from build123d import *

# Parameters (mm, degrees)
BOSS_EXTRUDE1_DEPTH     = 38.1
SKETCH2_W               = 25.4
SKETCH2_H               = 31.75
CUT_EXTRUDE1_DEPTH      = 88.9
CUT_EXTRUDE2_REACH      = 133.37
SKETCH3_W               = 25.4
SKETCH3_H               = 31.75
CUT_EXTRUDE3_START      = -62.861793
SKETCH4_W               = 75
SKETCH4_H               = 31.75
CUT_EXTRUDE3_DEPTH      = 28.575
FILLET4_R               = 20
CUT_EXTRUDE8_DEPTH      = 131.484388453
CUT_EXTRUDE8_DEPTH_BACK = 131.484388453
SKETCH8_R               = 6.35
BOSS_EXTRUDE2_DEPTH     = 3.175
CUT_EXTRUDE10_REACH     = 133.37
SKETCH35_R              = 3.175
CUT_EXTRUDE11_REACH     = 133.37
SKETCH36_R              = 3.175
FILLET8_R               = 5
CHAMFER1_SIZE           = 10
CHAMFER1_SIZE_2         = 7.071067812
CUT_EXTRUDE12_REACH     = 133.37
SKETCH37_R              = 3.175


with BuildPart() as part:
    # Sketch1 → Boss-Extrude1 (new body)
    with BuildSketch(Plane(origin=(0, 0, 0), x_dir=(1, 0, 0), z_dir=(0, 1, 0))):
        Polygon((0, 0), (-88.9, 0), (-88.9, 88.9), (-57.15, 88.9), (-57.15, 31.75), (0, 31.75), align=None)
    extrude(amount=BOSS_EXTRUDE1_DEPTH)

    # Sketch2 → Cut-Extrude1 (cut)
    with BuildSketch(Plane(origin=(0, 0, 0), x_dir=(0, 0, -1), z_dir=(1, 0, 0))):
        with Locations((15.875, 19.05)):
            Rectangle(SKETCH2_W, SKETCH2_H)
    extrude(amount=-CUT_EXTRUDE1_DEPTH, mode=Mode.SUBTRACT)

    # Cut-Extrude2: up to this face of the body (flat: up to its plane)
    cut_extrude2_end = Plane(part.part.faces().sort_by_distance((-44.45, 19.05, 0))[0])
    # Sketch3 → Cut-Extrude2 (cut, up to the picked face)
    with BuildSketch(Plane(origin=(0, 0, -88.9), x_dir=(-1, 0, 0), z_dir=(0, 0, -1)), mode=Mode.PRIVATE) as cut_extrude2_sk1:
        with Locations((73.025, 19.05)):
            Rectangle(SKETCH3_W, SKETCH3_H)
    cut_extrude2_tool1 = split(extrude(cut_extrude2_sk1.sketch, amount=-CUT_EXTRUDE2_REACH, mode=Mode.PRIVATE), bisect_by=cut_extrude2_end, keep=Keep.BOTH, mode=Mode.PRIVATE)
    add(cut_extrude2_tool1.solids().sort_by(Axis((-73.025, 19.05, -88.9), (0, 0, 1)))[0], mode=Mode.SUBTRACT)

    # Sketch4 → Cut-Extrude3 (cut)
    with BuildSketch(Plane(origin=(0, 0, 0), x_dir=(-0.7071067811865475, 0, -0.7071067811865476), z_dir=(0.7071067811865476, 0, -0.7071067811865475)).offset(CUT_EXTRUDE3_START)):
        with Locations((62.861792847, 19.05)):
            Rectangle(SKETCH4_W, SKETCH4_H)
    extrude(amount=CUT_EXTRUDE3_DEPTH, mode=Mode.SUBTRACT)

    # Fillet4
    fillet4_edges = [part.edges().sort_by_distance(p)[0] for p in [
        (-88.9, 36.5125, 0),
        (-88.9, 1.5875, 0),
    ]]
    fillet(fillet4_edges, radius=FILLET4_R)

    # Sketch8 → Cut-Extrude8 (cut, two sides: drawn at the far end of the back side and taken through both)
    with BuildSketch(Plane.XZ.offset(-34.925).offset(-CUT_EXTRUDE8_DEPTH_BACK)):
        with Locations(Location((-73.476280605, -15.423719395, 0), (0, 0, 270))):
            Circle(SKETCH8_R)
    extrude(amount=CUT_EXTRUDE8_DEPTH + CUT_EXTRUDE8_DEPTH_BACK, mode=Mode.SUBTRACT)

    # Sketch29 → Boss-Extrude2 (add)
    with BuildSketch(Plane(origin=(0, 38.1, 0), x_dir=(1, 0, 0), z_dir=(0, 1, 0))):
        Polygon((-57.15, 88.9), (0, 31.75), (-57.15, 31.75), align=None)
    boss_extrude2 = extrude(amount=-BOSS_EXTRUDE2_DEPTH)

    # Cut-Extrude10: up to this face of the body (flat: up to its plane)
    cut_extrude10_end = Plane(part.part.faces().sort_by_distance((-57.15, 17.4625, -60.325))[0])
    # Sketch35 → Cut-Extrude10 (cut, up to the picked face)
    with BuildSketch(Plane.ZY.offset(88.9), mode=Mode.PRIVATE) as cut_extrude10_sk1:
        with Locations((-78.65, 19.05)):
            Circle(SKETCH35_R)
    cut_extrude10_tool1 = split(extrude(cut_extrude10_sk1.sketch, amount=-CUT_EXTRUDE10_REACH, mode=Mode.PRIVATE), bisect_by=cut_extrude10_end, keep=Keep.BOTH, mode=Mode.PRIVATE)
    add(cut_extrude10_tool1.solids().sort_by(Axis((-88.9, 19.05, -78.65), (1, 0, 0)))[0], mode=Mode.SUBTRACT)

    # Cut-Extrude11: up to this face of the body (flat: up to its plane)
    cut_extrude11_end = Plane(part.part.faces().sort_by_distance((-28.575, 17.4625, -31.75))[0])
    # Sketch36 → Cut-Extrude11 (cut, up to the picked face)
    with BuildSketch(Plane.XY, mode=Mode.PRIVATE) as cut_extrude11_sk1:
        with Locations((-10.25, 19.05)):
            Circle(SKETCH36_R)
    cut_extrude11_tool1 = split(extrude(cut_extrude11_sk1.sketch, amount=-CUT_EXTRUDE11_REACH, mode=Mode.PRIVATE), bisect_by=cut_extrude11_end, keep=Keep.BOTH, mode=Mode.PRIVATE)
    add(cut_extrude11_tool1.solids().sort_by(Axis((-10.25, 19.05, 0), (0, 0, -1)))[0], mode=Mode.SUBTRACT)

    # Mirror1: Boss-Extrude2 across plane
    add(boss_extrude2.mirror(Plane(origin=(0, 19.05, 0), x_dir=(0, 0, 1), z_dir=(0, -1, 0))))

    # Fillet8
    fillet8_edges = [part.edges().sort_by_distance(p)[0] for p in [
        (-57.15, 19.05, -31.75),
        (-60.325, 19.05, -28.575),
    ]]
    fillet(fillet8_edges, radius=FILLET8_R)

    # Chamfer1
    # the kernel refuses this chamfer: 10, 7.071067812 mm, written as the material it takes off along each edge
    with BuildSketch(Plane(origin=(-51.663847671, 3.175, -3.175), x_dir=(0.9996219169112968, 0, -0.027495876610586317), z_dir=(0, 1, 0)), Plane(origin=(-85.725, 34.925, -37.236152329), x_dir=(0.027495876610586317, 0, -0.9996219169112968), z_dir=(0, -1, 0))) as chamfer1_piece_1:
        Polygon((CHAMFER1_SIZE * 0.999621916911, -CHAMFER1_SIZE * 0.0274958766106), (CHAMFER1_SIZE_2 * 0.687396915252, -CHAMFER1_SIZE_2 * 0.726281956863), (0, 0), align=None)
    extrude(amount=31.75, mode=Mode.SUBTRACT)

    # Cut-Extrude12: up to this face of the body (flat: up to its plane)
    cut_extrude12_end = Plane(part.part.faces().sort_by_distance((-50.123943702, 38.1, -38.776056298))[0])
    # Sketch37 → Cut-Extrude12 (cut, up to the picked face)
    with BuildSketch(Plane.XZ, mode=Mode.PRIVATE) as cut_extrude12_sk1:
        with Locations(Location((-42.045384182, -46.854615818, 0), (0, 0, 270))):
            Circle(SKETCH37_R)
    cut_extrude12_tool1 = split(extrude(cut_extrude12_sk1.sketch, amount=-CUT_EXTRUDE12_REACH, mode=Mode.PRIVATE), bisect_by=cut_extrude12_end, keep=Keep.BOTH, mode=Mode.PRIVATE)
    add(cut_extrude12_tool1.solids().sort_by(Axis((-42.045384, 0, -46.854616), (0, 1, 0)))[0], mode=Mode.SUBTRACT)


solid = part.part
Geometry: final body of the model. Coordinates: model frame, mm. A direction names the side the tool comes from. Coordinates: 2 decimals unless noted, no trailing zeros. Order: outer loops, then holes, each group sorted by start corner. A loop starts at its lowest first (then second) coordinate and runs counter-clockwise, first axis right, second up. Notation, with made-up numbers: (47.5, -23) - (99.5, -23) arc R8 ccw to (99.5, -9) - close; hole circle Ø1 at (-33.75, 69.25). An arc over 180 degrees is marked (long way). Use one line per item in the form item = value.
1) Section A-A (z = -24.5). Return loops of the section in (x, y) (3 decimals).
Solutions:
outline = (-88.9, 0) - (0, 0) - (0, 3.175) - (-88.9, 3.175) - close; (-88.9, 34.925) - (0, 34.925) - (0, 38.1) - (-88.9, 38.1) - close
2) Mould query, pull axis Z, two halves, no side actions, for faces 4 (the face through (-43.23, 18.83, -1.61)), 5 (the face through (-28.98, 1.57, -60.73)), 6 (the face through (-54, 38.1, -35)). Classes: +Z half, -Z half, draft (parallel to the pull), parting line (faces both ways), or undercut.
Solutions:
face_4 = undercut
face_5 = -Z half
face_6 = draft
3) Section D-D (x = -10.25). Return loops of the section in (y, z) (3 decimals).
Solutions:
outline = (0, -42) - (3.175, -42) - (3.175, -31.75) - (15.875, -31.75) - (15.875, -28.575) - (3.175, -28.575) - (3.175, -3.175) - (15.875, -3.175) - (15.875, 0) - (0, 0) - close; (22.225, -31.75) - (34.925, -31.75) - (34.925, -42) - (38.1, -42) - (38.1, 0) - (22.225, 0) - (22.225, -3.175) - (34.925, -3.175) - (34.925, -28.575) - (22.225, -28.575) - close
4) Section B-B (x = -21.5). Return loops of the section in (y, z) (3 decimals), then the cut area to 3 significant figures.
Solutions:
outline = (0, -53.25) - (3.175, -53.25) - (3.175, -31.75) - (34.925, -31.75) - (34.925, -53.25) - (38.1, -53.25) - (38.1, 0) - (0, 0) - close; hole (3.175, -28.575) - (34.925, -28.575) - (34.925, -3.175) - (3.175, -3.175) - close
area = 540 mm^2
5) Pin query (flat end, axial travel): pin 1 (10 mm diameter, centred on y = 19.05, z = -78.65, fed in from +X); pin 2 (16 mm diameter, centred on x = -27, y = 25.5, fed in from -Z). Return the tip coordinate at first contact, or that it passes through.
Solutions:
pin_1 = -57.15
pin_2 = -31.75
6) Ray query, L1, parallel to Z at x = -41, y = 16 (3 decimals); L2, parallel to Y at x = -38, z = -36.5 (3 decimals); L3, parallel to X at y = 6, z = -64.5 (3 decimals). Return the intervals inside material, ascending.
Solutions:
L1 = -31.75 to -28.575, -3.175 to 0
L2 = 0 to 3.175, 34.925 to 38.1
L3 = -88.9 to -85.725, -60.325 to -57.15
7) Section C-C (y = 32.5). Return loops of the section in (x, z) (3 decimals), then the cut area to 3 significant figures.
Solutions:
outline = (-88.9, -88.9) - (-85.725, -88.9) - (-85.725, -47.236) - (-88.9, -44.061) - close; (-60.325, -88.9) - (-57.15, -88.9) - (-57.15, -36.75) arc R5 cw to (-52.15, -31.75) - (0, -31.75) - (0, -28.575) - (-55.325, -28.575) arc R5 ccw to (-60.325, -33.575) - close; (-44.839, 0) - (-41.664, -3.175) - (0, -3.175) - (0, 0) - close
area = 648 mm^2
8) Set-up query: faces 1 (the face through (-35, 34.925, -48)), 2 (the face through (-87.29, 19.27, -45.67)), 3 (the face through (-85.725, 19, -68)). Return all of +Z, -Z, +X, -X, +Y, -Y with unobstructed straight access to the full face (end or side cutting, diameter ignored); none if empty.
Solutions:
face_1 = -Z, +X
face_2 = +Z
face_3 = +Z, -Z
